Work out the finished part from the listing and answer in its coordinate system (mm). Face numbers are marked on the shaded views. A direction names the side the tool comes from. Give positions to 0.01 mm unless a question says otherwise; leave off trailing zeros. Loops run counter-clockwise (first coordinate to the right, second up) from the corner with the lowest first, then second, coordinate; pieces in that order, holes last. Notation, with made-up numbers: (50.5, 80) - (87.5, 80) arc R19 ccw to (87.5, 108) - close; hole circle Ø8 at (23, -12). An arc over 180 degrees is marked (long way). One line per item, written item: value.
from build123d import *

# Parameters (mm, degrees)
F0_R     = 4
F1_DEPTH = 15
F2_DEPTH = 3
F4_DEPTH = 3


with BuildPart() as f1:
    # F0 (on Front) → F1 (new body)
    with BuildSketch(Plane.XZ):
        Circle(F0_R)
        with BuildLine():
            ThreePointArc((0.3, 1.9773719933), (1.5165750888, 1.303840481), (2, 0))
            ThreePointArc((2, 0), (1.5165750888, -1.303840481), (0.3, -1.9773719933))
            Line((0.3, -1.9773719933), (0.3, -2.5))
            Line((0.3, -2.5), (-0.3, -2.5))
            Line((-0.3, -2.5), (-0.3, -1.9773719933))
            ThreePointArc((-0.3, -1.9773719933), (-2, 0), (-0.3, 1.9773719933))
            Line((-0.3, 1.9773719933), (-0.3, 2.5))
            Line((-0.3, 2.5), (0.3, 2.5))
            Line((0.3, 2.5), (0.3, 1.9773719933))
        make_face(mode=Mode.SUBTRACT)
        with BuildLine():
            ThreePointArc((0.3, -1.9773719933), (1.5165750888, -1.303840481), (2, 0))
            ThreePointArc((2, 0), (1.5165750888, 1.303840481), (0.3, 1.9773719933))
            Line((0.3, 1.9773719933), (0.3, -1.9773719933))
        make_face()
        with BuildLine():
            Line((-0.3, -1.9773719933), (-0.3, 1.9773719933))
            ThreePointArc((-0.3, 1.9773719933), (-2, 0), (-0.3, -1.9773719933))
        make_face()
        with BuildLine():
            Line((0.3, -1.9773719933), (0.3, 1.9773719933))
            ThreePointArc((0.3, 1.9773719933), (0, 2), (-0.3, 1.9773719933))
            Line((-0.3, 1.9773719933), (-0.3, -1.9773719933))
            ThreePointArc((-0.3, -1.9773719933), (0, -2), (0.3, -1.9773719933))
        make_face()
        with BuildLine():
            ThreePointArc((-0.3, 1.9773719933), (0, 2), (0.3, 1.9773719933))
            Line((0.3, 1.9773719933), (0.3, 2.5))
            Line((0.3, 2.5), (-0.3, 2.5))
            Line((-0.3, 2.5), (-0.3, 1.9773719933))
        make_face()
        with BuildLine():
            Line((0.3, -2.5), (0.3, -1.9773719933))
            ThreePointArc((0.3, -1.9773719933), (0, -2), (-0.3, -1.9773719933))
            Line((-0.3, -1.9773719933), (-0.3, -2.5))
            Line((-0.3, -2.5), (0.3, -2.5))
        make_face()
    extrude(amount=-F1_DEPTH)

    # F0 (on Front) → F2 (cut)
    with BuildSketch(Plane.XZ):
        with BuildLine():
            Line((0.3, -1.9773719933), (0.3, 1.9773719933))
            ThreePointArc((0.3, 1.9773719933), (0, 2), (-0.3, 1.9773719933))
            Line((-0.3, 1.9773719933), (-0.3, -1.9773719933))
            ThreePointArc((-0.3, -1.9773719933), (0, -2), (0.3, -1.9773719933))
        make_face()
        with BuildLine():
            ThreePointArc((0.3, -1.9773719933), (1.5165750888, -1.303840481), (2, 0))
            ThreePointArc((2, 0), (1.5165750888, 1.303840481), (0.3, 1.9773719933))
            Line((0.3, 1.9773719933), (0.3, -1.9773719933))
        make_face()
        with BuildLine():
            ThreePointArc((-0.3, 1.9773719933), (0, 2), (0.3, 1.9773719933))
            Line((0.3, 1.9773719933), (0.3, 2.5))
            Line((0.3, 2.5), (-0.3, 2.5))
            Line((-0.3, 2.5), (-0.3, 1.9773719933))
        make_face()
        with BuildLine():
            Line((-0.3, -1.9773719933), (-0.3, 1.9773719933))
            ThreePointArc((-0.3, 1.9773719933), (-2, 0), (-0.3, -1.9773719933))
        make_face()
        with BuildLine():
            Line((0.3, -2.5), (0.3, -1.9773719933))
            ThreePointArc((0.3, -1.9773719933), (0, -2), (-0.3, -1.9773719933))
            Line((-0.3, -1.9773719933), (-0.3, -2.5))
            Line((-0.3, -2.5), (0.3, -2.5))
        make_face()
    extrude(amount=-F2_DEPTH, mode=Mode.SUBTRACT)

    # F3 (on face) → F4 (join)
    with BuildSketch(Plane(origin=(0, 15, 0), x_dir=(-1, 0, 0), z_dir=(0, 1, 0))):
        with BuildLine():
            Line((-0.25, -1.4282856857), (-0.25, 1.4282856857))
            ThreePointArc((-0.25, 1.4282856857), (-1.45, 0), (-0.25, -1.4282856857))
        make_face()
        with BuildLine():
            Line((0.25, -1.4282856857), (0.25, 1.4282856857))
            ThreePointArc((0.25, 1.4282856857), (0, 1.45), (-0.25, 1.4282856857))
            Line((-0.25, 1.4282856857), (-0.25, -1.4282856857))
            ThreePointArc((-0.25, -1.4282856857), (0, -1.45), (0.25, -1.4282856857))
        make_face()
        with BuildLine():
            ThreePointArc((0.25, -1.4282856857), (1.1101801656, -0.9327379053), (1.45, 0))
            ThreePointArc((1.45, 0), (1.1101801656, 0.9327379053), (0.25, 1.4282856857))
            Line((0.25, 1.4282856857), (0.25, -1.4282856857))
        make_face()
        with BuildLine():
            ThreePointArc((-0.25, 1.4282856857), (0, 1.45), (0.25, 1.4282856857))
            Line((0.25, 1.4282856857), (0.25, 2.45))
            Line((0.25, 2.45), (-0.25, 2.45))
            Line((-0.25, 2.45), (-0.25, 1.4282856857))
        make_face()
        with BuildLine():
            Line((0.25, -2.45), (0.25, -1.4282856857))
            ThreePointArc((0.25, -1.4282856857), (0, -1.45), (-0.25, -1.4282856857))
            Line((-0.25, -1.4282856857), (-0.25, -2.45))
            Line((-0.25, -2.45), (0.25, -2.45))
        make_face()
    extrude(amount=F4_DEPTH)


solid = f1.part
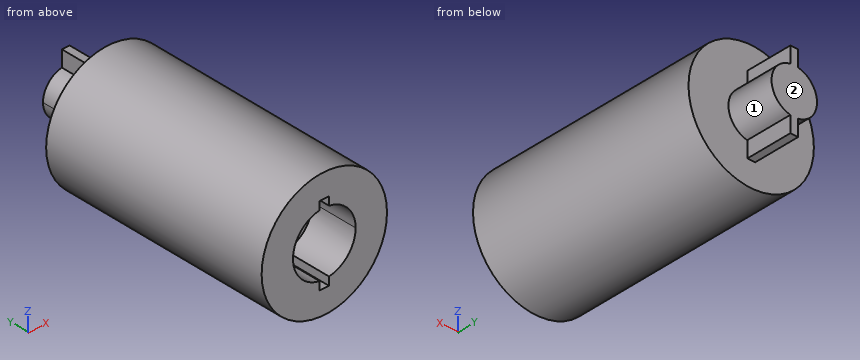
1. Flat-ended cylindrical pins translate along their axes: pin 1 Ø0.6 at (y, z) = (2, 2.5) entering from -X; pin 2 Ø0.8 at (y, z) = (17, 2) entering from -X; pin 3 Ø0.6 at (x, y) = (0, 16) entering from +Z. Find the tip coordinate at first contact, or state that the pin passes through.
Output:
pin 1: stops at x = -3.34
pin 2: stops at x = -0.25
pin 3: stops at z = 2.45
2. Section B-B (x = 0) is taken. Write down the section's boundary in (y, z).
Output:
outline: (0, -4) - (15, -4) - (15, -2.45) - (18, -2.45) - (18, 2.45) - (15, 2.45) - (15, 4) - (0, 4) - (0, 2.5) - (3, 2.5) - (3, -2.5) - (0, -2.5) - close
3. Section D-D (z = -0.5) is taken. Write down the section's boundary in (x, y), and give its area (3 significant figures).
Output:
outline: (-3.97, 0) - (-1.94, 0) - (-1.94, 3) - (1.94, 3) - (1.94, 0) - (3.97, 0) - (3.97, 15) - (1.36, 15) - (1.36, 18) - (-1.36, 18) - (-1.36, 15) - (-3.97, 15) - close
area: 116 mm²
4. Section C-C (y = 16) is taken. Write down the section's boundary in (x, z).
Output:
outline: (-0.25, -2.45) - (0.25, -2.45) - (0.25, -1.43) arc R1.45 ccw to (0.25, 1.43) - (0.25, 2.45) - (-0.25, 2.45) - (-0.25, 1.43) arc R1.45 ccw to (-0.25, -1.43) - close
5. Find the intervals of material crossed by line 1 along Y through (x, z) = (2.5, 3); line 2 along Z through (x, y) = (1.25, 2.75); line 3 along X through (y, z) = (2.75, 0.5), in increasing order.
Output:
line 1: y = 0 to 15
line 2: z = -3.8 to -1.56, 1.56 to 3.8
line 3: x = -3.97 to -1.94, 1.94 to 3.97
6. Section A-A (y = 1.5) is taken. Write down the section's boundary in (x, z).
Output:
outline: circle Ø8 at (0, 0); hole (-0.3, -2.5) - (0.3, -2.5) - (0.3, -1.98) arc R2 ccw to (0.3, 1.98) - (0.3, 2.5) - (-0.3, 2.5) - (-0.3, 1.98) arc R2 ccw to (-0.3, -1.98) - close
7. For the marked faces 1 and 2, determine the directions among +Z, -Z, +X, -X, +Y, -Y from which every point of the face is accessible in a straight line to the end or side of a thin tool.
Output:
face 1: +X, +Y
face 2: +Z, -Z, +X, -X, +Y
